Input: part model. Units: mm. Frame: model coordinates. Face numbers are marked on the shaded views. A direction names the side the tool comes from. Give positions to 0.01 mm unless a question says otherwise; leave off trailing zeros. Loops run counter-clockwise (first coordinate to the right, second up) from the corner with the lowest first, then second, coordinate; pieces in that order, holes last. Notation, with made-up numbers: (-3.5, 21.5) -> (35.5, 21.5) arc R8 cw to (35.5, 25.5) -> close; hole circle Ø10 at (46.5, 63.25). An arc over 180 degrees is marked (long way). One line per question, with ' | ' between items.
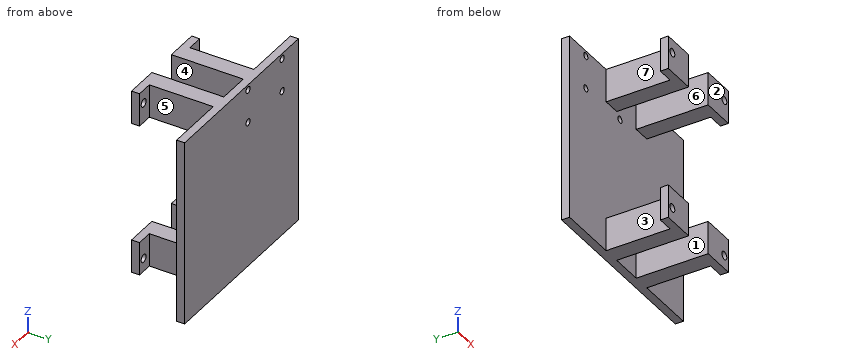
from build123d import *

# Parameters (mm, degrees)
EXTRUDE_1_DEPTH     = 35
SKETCH_2_W          = 45
SKETCH_2_H          = 27
CUT_EXTRUDE_1_DEPTH = 35
SKETCH_3_W          = 12
SKETCH_3_H          = 27
CUT_EXTRUDE_2_DEPTH = 40
SKETCH_4_R          = 1.5
CUT_EXTRUDE_3_DEPTH = 19
SKETCH_5_R          = 1.25
CUT_EXTRUDE_4_DEPTH = 5


with BuildPart() as part:
    # 草圖1 → 填料-伸長1 (new, symmetric)
    with BuildSketch(Plane.XY):
        Polygon((-18.5, 0), (-18.5, 3), (-12.5, 3), (-12.5, 27), (-35, 27), (-35, 30), (35, 30), (35, 27), (12.5, 27), (12.5, 3), (18.5, 3), (18.5, 0), align=None)
    extrude(amount=EXTRUDE_1_DEPTH, both=True)

    # 草圖2 → 除料-伸長1 (cut, symmetric)
    with BuildSketch(Plane(origin=(0, 0, 0), x_dir=(0, 0, -1), z_dir=(1, 0, 0))):
        with Locations((0, 13.5)):
            Rectangle(SKETCH_2_W, SKETCH_2_H)
    extrude(amount=CUT_EXTRUDE_1_DEPTH, both=True, mode=Mode.SUBTRACT)

    # 草圖3 → 除料-伸長2 (cut, symmetric)
    with BuildSketch(Plane.XY):
        with Locations((0, 13.5)):
            Rectangle(SKETCH_3_W, SKETCH_3_H)
    extrude(amount=CUT_EXTRUDE_2_DEPTH, both=True, mode=Mode.SUBTRACT)

    # 草圖4 → 除料-伸長3 (cut)
    with BuildSketch(Plane(origin=(0, 0, 0), x_dir=(1, 0, 0), z_dir=(0, 1, 0))):
        with Locations(Location((-16, -30, 0), (0, 0, 90))):
            Circle(SKETCH_4_R)
        with Locations(Location((16, -30, 0), (0, 0, 90))):
            Circle(SKETCH_4_R)
        with Locations(Location((16, 30, 0), (0, 0, 90))):
            Circle(SKETCH_4_R)
        with Locations(Location((-16, 30, 0), (0, 0, 90))):
            Circle(SKETCH_4_R)
    extrude(amount=CUT_EXTRUDE_3_DEPTH, mode=Mode.SUBTRACT)

    # 草圖5 → 除料-伸長4 (cut, symmetric)
    with BuildSketch(Plane(origin=(0, 30, 0), x_dir=(1, 0, 0), z_dir=(0, 1, 0))):
        with Locations(Location((-4, -20.5, 0), (0, 0, 180))):
            Circle(SKETCH_5_R)
        with Locations(Location((-4, -33, 0), (0, 0, 180))):
            Circle(SKETCH_5_R)
        with Locations(Location((-25, -33, 0), (0, 0, 180))):
            Circle(SKETCH_5_R)
        with Locations(Location((-25, -20.5, 0), (0, 0, 180))):
            Circle(SKETCH_5_R)
    extrude(amount=CUT_EXTRUDE_4_DEPTH, both=True, mode=Mode.SUBTRACT)


solid = part.part
1. Section query B-B (y = 9.25). Output: boundary loops of the cut face in (x, z), then the cut area to 3 significant figures.
Determined:
outline: (-12.5, -35) -> (-6, -35) -> (-6, -22.5) -> (-12.5, -22.5) -> close; (-12.5, 22.5) -> (-6, 22.5) -> (-6, 35) -> (-12.5, 35) -> close; (6, -35) -> (12.5, -35) -> (12.5, -22.5) -> (6, -22.5) -> close; (6, 22.5) -> (12.5, 22.5) -> (12.5, 35) -> (6, 35) -> close | area: 325 mm2
2. Section query D-D (x = -16). Output: boundary loops of the cut face in (y, z).
Determined:
outline: (0, -35) -> (3, -35) -> (3, -31.5) -> (0, -31.5) -> close; (0, -28.5) -> (3, -28.5) -> (3, -22.5) -> (0, -22.5) -> close; (0, 22.5) -> (3, 22.5) -> (3, 28.5) -> (0, 28.5) -> close; (0, 31.5) -> (3, 31.5) -> (3, 35) -> (0, 35) -> close; (27, -35) -> (30, -35) -> (30, 35) -> (27, 35) -> close
3. Reachability of the marked faces 5, 6 and 7 from +Z, -Z, +X, -X, +Y, -Y: full face, straight path, thin tool, end or side. Return the list, or none.
Determined:
face 5: +Z, -Z, +X | face 6: +Z, -Z, -Y | face 7: +Z, -Z, -X
4. Ray query, line 1 along Z through (x, y) = (-16, 1.2); line 2 along Z through (x, y) = (-25, 28.2); line 3 along X through (y, z) = (1.5, 30). Return the intervals inside material, ascending. Write a range as from..to.
Determined:
line 1: z = -35..-31.5, -28.5..-22.5, 22.5..28.5, 31.5..35 | line 2: z = -35..19.25, 21.75..31.75, 34.25..35 | line 3: x = -18.5..-17.5, -14.5..-6, 6..14.5, 17.5..18.5
5. Pull-direction query (X, two-part tool) for the marked faces 1, 2, 3 and 4; classes: pulls with the +X half, pulls with the -X half, needs draft (parallel to the pull), parting line crosses it, or undercut.
Determined:
face 1: undercut | face 2: needs draft | face 3: pulls with the -X half | face 4: undercut
6. Pin query (flat end, axial travel): P1, Ø2.5, axis at y = 1.5, z = 31, coming from the -X side; P2, Ø0.9, axis at y = 1, z = -31, coming from the +X side; P3, Ø2.5, axis at x = -16, z = -30, coming from the -Y side. Return the tip coordinate at first contact, or that it passes through.
Determined:
P1: stops at x = -18.5 | P2: stops at x = 18.5 | P3: stops at y = 27
7. Section query C-C (x = -25). Output: boundary loops of the cut face in (y, z).
Determined:
outline: (27, -35) -> (30, -35) -> (30, 19.25) -> (27, 19.25) -> close; (27, 21.75) -> (30, 21.75) -> (30, 31.75) -> (27, 31.75) -> close; (27, 34.25) -> (30, 34.25) -> (30, 35) -> (27, 35) -> close
8. Section query A-A (z = 33). Output: boundary loops of the cut face in (x, y), then the cut area to 3 significant figures.
Determined:
outline: (-35, 27) -> (-26.25, 27) -> (-26.25, 30) -> (-35, 30) -> close; (-23.75, 27) -> (-12.5, 27) -> (-12.5, 3) -> (-18.5, 3) -> (-18.5, 0) -> (-6, 0) -> (-6, 27) -> (-5.25, 27) -> (-5.25, 30) -> (-23.75, 30) -> close; (-2.75, 27) -> (6, 27) -> (6, 0) -> (18.5, 0) -> (18.5, 3) -> (12.5, 3) -> (12.5, 27) -> (35, 27) -> (35, 30) -> (-2.75, 30) -> close | area: 582 mm2
